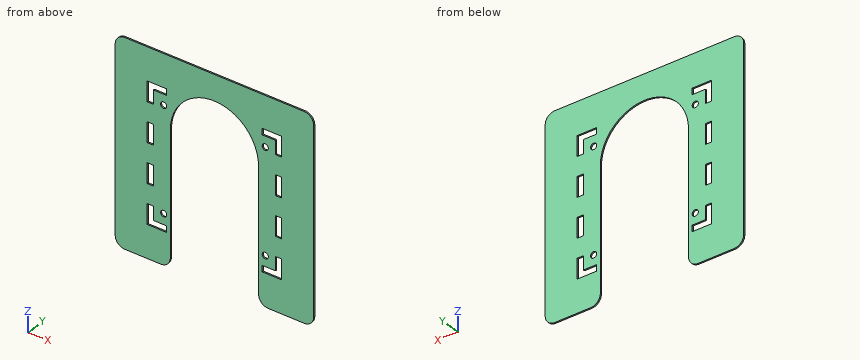
from build123d import *

# Parameters (mm, degrees)
SKETCH1_R           = 1.6
BOSS_EXTRUDE1_DEPTH = 0.75
SKETCH3_W           = 3.2
SKETCH3_H           = 10.21670071
SKETCH3_H_2         = 10.216700711
CUT_EXTRUDE1_DEPTH  = 1.75


with BuildPart() as part:
    # Sketch1 → Boss-Extrude1 (new body)
    with BuildSketch(Plane(origin=(0, 0, 0), x_dir=(1, 0, 0), z_dir=(0, 1, 0))):
        with BuildLine():
            Line((51.872217102, -34.901443346), (51.872217102, 58.842990858))
            ThreePointArc((51.872217102, 58.842990858), (50.407751008, 62.378524764), (46.872217102, 63.842990858))
            Line((46.872217102, 63.842990858), (28.058452488, 63.842990858))
            ThreePointArc((28.058452488, 63.842990858), (24.522918582, 62.378524764), (23.058452488, 58.842990858))
            Line((23.058452488, 58.842990858), (23.058452488, -3.842990858))
            ThreePointArc((23.058452488, -3.842990858), (0, -26.901443346), (-23.058452488, -3.842990858))
            Line((-23.058452488, -3.842990858), (-23.058452488, 58.842990858))
            ThreePointArc((-23.058452488, 58.842990858), (-24.522918582, 62.378524764), (-28.058452488, 63.842990858))
            Line((-28.058452488, 63.842990858), (-46.872217102, 63.842990858))
            ThreePointArc((-46.872217102, 63.842990858), (-50.407751008, 62.378524764), (-51.872217102, 58.842990858))
            Line((-51.872217102, 58.842990858), (-51.872217102, -34.901443346))
            ThreePointArc((-51.872217102, -34.901443346), (-50.407751008, -38.436977252), (-46.872217102, -39.901443346))
            Line((-46.872217102, -39.901443346), (46.872217102, -39.901443346))
            ThreePointArc((46.872217102, -39.901443346), (50.407751008, -38.436977252), (51.872217102, -34.901443346))
        make_face()
        with Locations((26.558452488, -14.587678732)):
            Circle(SKETCH1_R, mode=Mode.SUBTRACT)
        with Locations((-26.558452488, -14.587678732)):
            Circle(SKETCH1_R, mode=Mode.SUBTRACT)
        with Locations((26.558452488, 38.529226244)):
            Circle(SKETCH1_R, mode=Mode.SUBTRACT)
        with Locations((-26.558452488, 38.529226244)):
            Circle(SKETCH1_R, mode=Mode.SUBTRACT)
    extrude(amount=-BOSS_EXTRUDE1_DEPTH)

    # Sketch3 → Cut-Extrude1 (cut, through all)
    with BuildSketch(Plane(origin=(0, 0, 0), x_dir=(1, 0, 0), z_dir=(0, 1, 0))):
        with Locations((33.558452488, 1.954073045)):
            Rectangle(SKETCH3_W, SKETCH3_H)
        Polygon((35.158452488, 36.912525533), (35.158452488, 47.129226244), (24.941751777, 47.129226244), (24.941751777, 43.929226244), (31.958452488, 43.929226244), (31.958452488, 36.912525533), align=None)
        with Locations((33.558452488, 21.987474467)):
            Rectangle(SKETCH3_W, SKETCH3_H_2)
        with Locations((-33.558452488, 21.987474467)):
            Rectangle(SKETCH3_W, SKETCH3_H_2)
        Polygon((-31.958452488, 36.912525533), (-31.958452488, 43.929226244), (-24.941751777, 43.929226244), (-24.941751777, 47.129226244), (-35.158452488, 47.129226244), (-35.158452488, 36.912525533), align=None)
        Polygon((31.958452488, -12.970978021), (31.958452488, -19.987678732), (24.941751777, -19.987678732), (24.941751777, -23.187678732), (35.158452488, -23.187678732), (35.158452488, -12.970978021), align=None)
        Polygon((-35.158452488, -12.970978021), (-35.158452488, -23.187678732), (-24.941751777, -23.187678732), (-24.941751777, -19.987678732), (-31.958452488, -19.987678732), (-31.958452488, -12.970978021), align=None)
        with Locations((-33.558452488, 1.954073045)):
            Rectangle(SKETCH3_W, SKETCH3_H)
    extrude(amount=-CUT_EXTRUDE1_DEPTH, mode=Mode.SUBTRACT)


solid = part.part
For this review, take the finished solid that the model builds, in its own axes (mm). Coordinates: 2 decimals unless noted, no trailing zeros. Loops run counter-clockwise (first coordinate to the right, second up) from the corner with the lowest first, then second, coordinate; pieces in that order, holes last. Notation, with made-up numbers: (-26, 46) - (-18, 46) arc R10 cw to (-18, 56) - close; hole circle Ø10 at (-37.75, 52). An arc over 180 degrees is marked (long way). Use a Markdown table: item, result. Add a question column.
Item 1: We need section D-D (y = -0.4). Give the number of separate pieces and of enclosed holes in the cut face, and give its area (3 significant figures).
Item 2: We need section A-A (z = -18.5). Give the boundary of the cut face in (x, y).
Item 3: We need section C-C (x = 0). Give the boundary of the cut face in (y, z).
Item 4: We need section B-B (z = 18.5). Give the boundary of the cut face in (x, y).
Item 5: For line 1 (X direction, y = -0.4, z = -45.5); line 2 (X direction, y = -0.65, z = -15.5); line 3 (X direction, y = -0.15, z = 1), list the stretches that pass through material, from the lowest coordinate up.
Results list:
| question | item | result |
|---|---|---|
| 1 | separate pieces | 1 |
| 1 | enclosed holes | 12 |
| 1 | area | 6,390 mm^2 |
| 2 | outline | (-51.87, -0.75) - (-35.16, -0.75) - (-35.16, 0) - (-51.87, 0) - close; (-31.96, -0.75) - (-23.06, -0.75) - (-23.06, 0) - (-31.96, 0) - close; (23.06, -0.75) - (31.96, -0.75) - (31.96, 0) - (23.06, 0) - close; (35.16, -0.75) - (51.87, -0.75) - (51.87, 0) - (35.16, 0) - close |
| 3 | outline | (-0.75, 26.9) - (0, 26.9) - (0, 39.9) - (-0.75, 39.9) - close |
| 4 | outline | (-51.87, -0.75) - (-35.16, -0.75) - (-35.16, 0) - (-51.87, 0) - close; (-31.96, -0.75) - (-17.8, -0.75) - (-17.8, 0) - (-31.96, 0) - close; (17.8, -0.75) - (31.96, -0.75) - (31.96, 0) - (17.8, 0) - close; (35.16, -0.75) - (51.87, -0.75) - (51.87, 0) - (35.16, 0) - close |
| 5 | line 1 | x = -51.87 to -35.16, -24.94 to -23.06, 23.06 to 24.94, 35.16 to 51.87 |
| 5 | line 2 | x = -51.87 to -23.06, 23.06 to 51.87 |
| 5 | line 3 | x = -51.87 to -35.16, -31.96 to -23.06, 23.06 to 31.96, 35.16 to 51.87 |
